Geometry: see drawing. Coordinates: mm, zero at the bounding-box minimum. Give positions to 0.01 mm unless a question says otherwise; leave off trailing zeros. Write each loop counter-clockwise with the first axis right and the second up, starting at its lowest first coordinate (ties: lowest second). Pieces come first, ordered by that corner, then holes. Notation, with made-up numbers: M 26,32.25 L 31,32.25 A18 ccw 31,44.25 Z; hole C -21,-4 d11. An arc over 180 degrees is marked long. Use a Markdown table: item, result. Add a question column.
(1) Material intervals for L1, parallel to Y at x = 3.4, z = 98.5 (3 decimals); L2, parallel to Z at x = 2.55, y = 57; L3, parallel to Z at x = 2.85, y = 40.5, sorted ascending.
(2) Pin query (flat end, axial travel): pin 1 Ø2.5 at (y, z) = (34.925, 98.5) entering from +X. Return the tip coordinate at first contact, or that it passes through.
(3) Cut plane A-A (z = 12.7). Output: boundary loops of the cut face in (x, y), plus the area to 3 significant figures.
(4) Cut plane B-B (z = 98.5). Output: boundary loops of the cut face in (x, y) (3 decimals).
(5) Cut plane C-C (y = 61.5). Output: boundary loops of the cut face in (x, z).
(6) Cut plane D-D (x = 3.55). State how many separate pieces and enclosed holes the cut face has, plus the area to 3 significant figures.
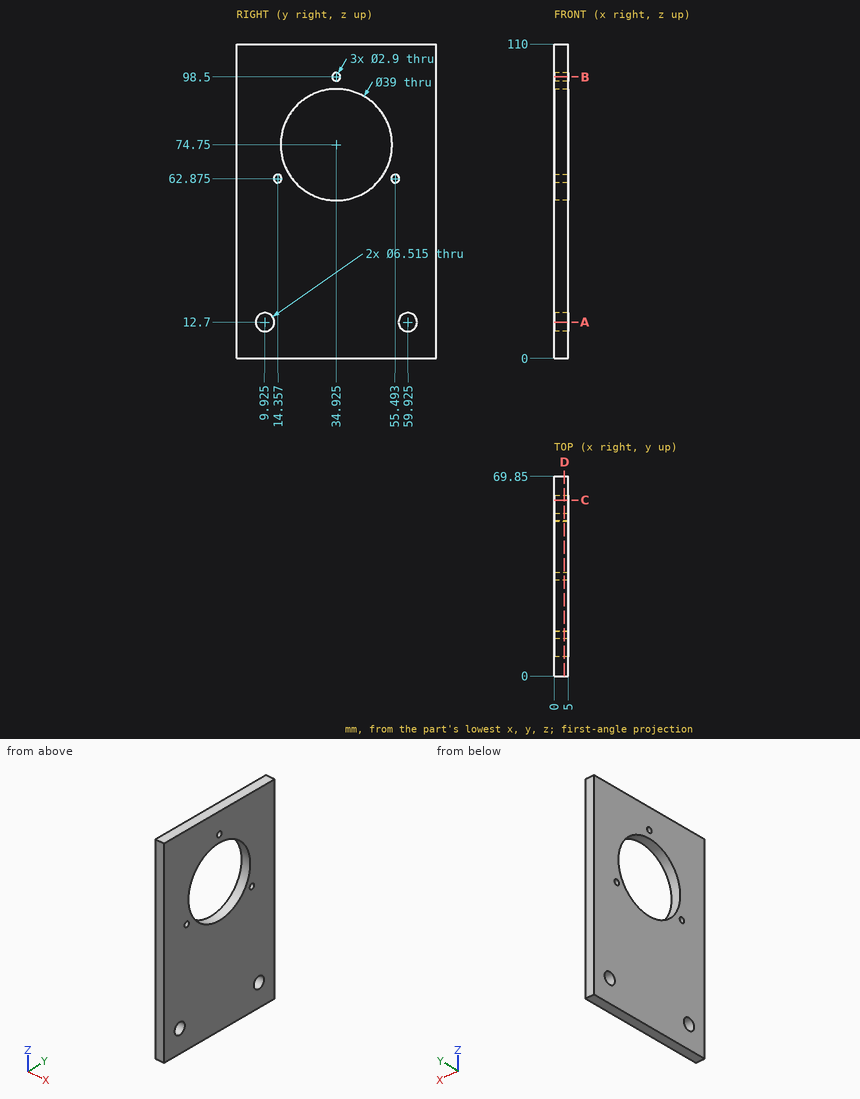
Answer list:
| question | item | result |
|---|---|---|
| 1 | L1 | 0 to 33.475, 36.375 to 69.85 |
| 1 | L2 | 0 to 11.27, 14.13 to 110 |
| 1 | L3 | 0 to 56.06, 93.44 to 110 |
| 2 | pin 1 | through |
| 3 | outline | M 0,0 L 5,0 L 5,6.67 L 0,6.67 Z; M 0,13.18 L 5,13.18 L 5,56.67 L 0,56.67 Z; M 0,63.18 L 5,63.18 L 5,69.85 L 0,69.85 Z |
| 3 | area | 284 mm² |
| 4 | outline | M 0,0 L 5,0 L 5,33.475 L 0,33.475 Z; M 0,36.375 L 5,36.375 L 5,69.85 L 0,69.85 Z |
| 5 | outline | M 0,0 L 5,0 L 5,9.85 L 0,9.85 Z; M 0,15.55 L 5,15.55 L 5,110 L 0,110 Z |
| 6 | separate pieces | 1 |
| 6 | enclosed holes | 6 |
| 6 | area | 6,400 mm² |
